Autodesk Inventor part; units mm, degrees
ref_plane "YZ Plane" through (0, 0, 0) normal (1, 0, 0) x (0, 1, 0)
ref_plane "XZ Plane" through (0, 0, 0) normal (0, 1, 0) x (-1, 0, 0)
ref_plane "XY Plane" through (0, 0, 0) normal (0, 0, 1) x (1, 0, 0)
sketch "Sketch1" plane through (0, 0, 0) normal (0, 1, 0) x (-1, 0, 0)
  circle A0 centre (0, 0) radius 32.5
  circle A1 centre (0, 0) radius 25
  circle A2 centre (17.3494, -18) radius 5
  circle A3 centre (18, 17.3494) radius 5
  circle A4 centre (-17.3494, 18) radius 5
  circle A5 centre (-18, -17.3494) radius 5
  line L0 (6, -18) -> (-6, -18) construction
  line L1 (6, -15.7639) -> (-6, -15.7639)
  line L2 (-6, -20.2361) -> (6, -20.2361)
  arc A6 (6, -20.2361) -> (6, -15.7639) centre (6, -18) ccw
  arc A7 (-6, -15.7639) -> (-6, -20.2361) centre (-6, -18) ccw
  line L3 (-25, 0) -> (25, 0) construction
  line L4 (6, 15.7639) -> (-6, 15.7639)
  line L5 (-6, 20.2361) -> (6, 20.2361)
  arc A8 (6, 15.7639) -> (6, 20.2361) centre (6, 18) ccw
  arc A9 (-6, 20.2361) -> (-6, 15.7639) centre (-6, 18) ccw
  circle A10 centre (0, 0) radius 37.5
  point P0 (0, -18)
  dimension "d0" = 65
  dimension "d1" = 50
  dimension "d2" = 10
  dimension "d5" = 360
  dimension "d7" = 35.3494
  dimension "d11" = 17.3494
  dimension "d12" = 11.3493
  dimension "d16" = 18
  dimension "d17" = 2.2361
  dimension "d18" = 18
  dimension "d19" = 75
extrude "Extrusion1" add sketch "Sketch1" against normal blind 6.5 contours A0 | A1 A2 A5 A4 A3
extrude "Extrusion2" add sketch "Sketch1" along normal blind 6.5 and the other way blind 6.5 contours A10
sketch "Sketch2" plane through (0, -6.5, 0) normal (0, -1, 0) x (1, 0, 0)
  line L0 (35, 5) -> (-35, 5)
  line L1 (-35, 5) -> (-35, -5)
  line L2 (-35, -5) -> (35, -5)
  line L3 (35, -5) -> (35, 5)
  line L4 (35, 5) -> (-35, -5) construction
  line L5 (-35, 5) -> (35, -5) construction
  point P0 (0, 0)
  dimension "d24" = 10
  dimension "d25" = 70
extrude "Extrusion3" cut sketch "Sketch2" against normal blind 5
extrude "Extrusion4" add sketch "Sketch1" along normal blind 6.5 contours A0 | A1 A2 A5 A4 A3
sketch "Sketch3" plane through (0, 6.5, 0) normal (0, 1, 0) x (1, 0, 0)
  line L0 (-26.5, -5.5) -> (26.5, -5.5)
  line L1 (26.5, -5.5) -> (26.5, 5.5)
  line L2 (26.5, 5.5) -> (-26.5, 5.5)
  line L3 (-26.5, 5.5) -> (-26.5, -5.5)
  line L4 (-26.5, -5.5) -> (26.5, 5.5) construction
  line L5 (26.5, -5.5) -> (-26.5, 5.5) construction
  point P0 (0, 0)
  dimension "d32" = 11
  dimension "d33" = 53
extrude "Extrusion5" cut sketch "Sketch3" against normal blind 3.5
properties part number "case_top"
Can you work these out from the model? Positions are in its coordinate system, mm. A direction names the side the tool comes from. Coordinates: 2 decimals unless noted, no trailing zeros. Write each loop counter-clockwise with the first axis right and the second up, starting at its lowest first coordinate (ties: lowest second). Pieces come first, ordered by that corner, then holes.
Q1. Imagine slicing it at C-C, the plane x = -30. List the corners of the cut face in (y, z) for me.
Results found:
outline: (-6.5, -22.5) - (6.5, -22.5) - (6.5, 22.5) - (-6.5, 22.5) - (-6.5, 5) - (-1.5, 5) - (-1.5, -5) - (-6.5, -5) - close
Q2. Imagine slicing it at A-A, the plane x = 0. List the corners of the cut face in (y, z) for me.
Results found:
outline: (-6.5, -37.5) - (6.5, -37.5) - (6.5, -20.24) - (-6.5, -20.24) - close; (-6.5, -15.76) - (6.5, -15.76) - (6.5, -5.5) - (3, -5.5) - (3, 5.5) - (6.5, 5.5) - (6.5, 15.76) - (-6.5, 15.76) - (-6.5, 5) - (-1.5, 5) - (-1.5, -5) - (-6.5, -5) - close; (-6.5, 20.24) - (6.5, 20.24) - (6.5, 37.5) - (-6.5, 37.5) - close
Q3. If we mould it in two halves opening along X, with no side actions, what happens to faces 1 (the face through (0, -4, -5)), 2 (the face through (-26.5, 5, 0)), 3 (the face through (4.88, -0.09, -37.18)), 4 (the face through (1, -6.5, -8))? For each: +X half, -X half, draft (parallel to the pull), parting line (faces both ways), or undercut.
Results found:
face 1: undercut
face 2: undercut
face 3: parting line
face 4: draft
Q4. Please list where these lines run through material, in increasing order: L1, parallel to Z at x = -0.5, y = -3; L2, parallel to X at y = 0.5, z = 18; L3, parallel to Z at x = 3, y = 2.
Results found:
L1: z = -37.5 to -20.24, -15.76 to -5, 5 to 15.76, 20.24 to 37.5
L2: x = -32.9 to -22.96, -13.04 to -8.24, 8.24 to 12.35, 22.35 to 32.9
L3: z = -37.38 to -20.24, -15.76 to 15.76, 20.24 to 37.38
Q5. Which directions (+Z, -Z, +X, -X, +Y, -Y) give clear straight access to the entire face, cutting with the end or side of a thin tool? Please do faces 5 (the face through (1, 6.5, -8)), 6 (the face through (0, 0, 20.236)), 7 (the face through (-35, -4, 0)), 8 (the face through (0, 3, 0)).
Results found:
face 5: +Z, -Z, +X, -X, +Y
face 6: +Y, -Y
face 7: -Y
face 8: +Y
Q6. Imagine slicing it at D-D, the plane z = 0. List the corners of the cut face in (x, y) for me, plus the area to 4 significant figures.
Results found:
outline: (-37.5, -6.5) - (-35, -6.5) - (-35, -1.5) - (35, -1.5) - (35, -6.5) - (37.5, -6.5) - (37.5, 6.5) - (26.5, 6.5) - (26.5, 3) - (-26.5, 3) - (-26.5, 6.5) - (-37.5, 6.5) - close
area: 439.5 mm2
Q7. Imagine slicing it at B-B, the plane y = -0.25. List the corners of the cut face in (x, z) for me, plus the area to 3 significant figures.
Results found:
outline: circle Ø75 at (0, 0); hole circle Ø10 at (-18, 17.35); hole circle Ø10 at (-17.35, -18); hole (-6, -20.24) - (6, -20.24) arc R2.24 ccw to (6, -15.76) - (-6, -15.76) arc R2.24 ccw to start; hole (-6, 15.76) - (6, 15.76) arc R2.24 ccw to (6, 20.24) - (-6, 20.24) arc R2.24 ccw to start; hole circle Ø10 at (17.35, 18); hole circle Ø10 at (18, -17.35)
area: 3,960 mm2
Q8. For P1, Ø9, axis at x = 17.35, z = 18, coming from the +Y side; P2, Ø3, axis at x = -5, z = -2.5, coming from the -Y side; P3, Ø4, axis at y = 4.5, z = -7.5, coming from the -X side; P4, Ø4, axis at x = -13, y = 5.5, coming from the -Z side, each with a flat end and sliding along its axis, tell me the tip position at first contact or that it passes through.
Results found:
P1: passes through
P2: stops at y = -1.5
P3: stops at x = -37.09
P4: stops at z = -35.85
